Here's how the part is built. I have some questions about the finished solid (model axes, mm). A direction names the side the tool comes from. Coordinates: 2 decimals unless noted, no trailing zeros. Write each loop counter-clockwise with the first axis right and the second up, starting at its lowest first coordinate (ties: lowest second). Pieces come first, ordered by that corner, then holes.
Item 1: Please list where these lines run through material, in increasing order: line 1 (X direction, y = 18, z = 37.65); line 2 (Y direction, x = 24, z = 36.85); line 3 (X direction, y = -13, z = 12.5).
Item 2: I want a section at B-B (z = 25.2). Please give me the cut outline in (x, y).
Item 3: If we mould it in two halves opening along Y, with no side actions, what happens to faces 4 (the face through (-23.8, 17.92, 34.63)), 5 (the face through (32.5, 0, 19)), 6 (the face through (-35.95, 0.78, 31.15))? For each: pulls with the +Y half, pulls with the -Y half, needs draft (parallel to the pull), parting line crosses it, or undercut.
Item 4: I want a section at A-A (y = 0). Please give me the cut outline in (x, z), and give its area (3 significant figures).
Item 5: For faces 1 (the face through (-25.19, -17.62, 37.35)), 2 (the face through (0, -32.5, 19)), 3 (the face through (-22, 15, 0)), which set-ups out of +Z, -Z, +X, -X, +Y, -Y let a thin tool reach every point of the face, with its end or its side?
Item 6: I want a section at D-D (y = -14.5). Please give me the cut outline in (x, z).
Item 7: I'm going to push flat-ended pins straight in: P1, Ø2, axis at x = -24, y = -18, coming from the -Z side; P2, Ø2, axis at x = -24, y = 18, coming from the +Z side; P3, Ø1.5, axis at x = 13, y = 5.5, coming from the -Z side. Where does each tip first touch, or does it pass through?
Item 8: I want a section at C-C (x = -5.5). Please give me the cut outline in (y, z).
from build123d import *

# Parameters (mm, degrees)
SCHIZZO1_W                   = 65
SCHIZZO1_H                   = 65
ESTRUSIONE_ESTRUSIONE1_DEPTH = 39.5
SCHIZZO14_R                  = 6
ESTRUSIONE_ESTRUSIONE2_DEPTH = 7
FORO_FILETTATO_M3_1_D        = 2.5
FORO_FILETTATO_M3_1_DEPTH    = 4.248924226
FORO_FILETTATO_M3_1_TIP      = 0.751075774


with BuildPart() as part:
    # Schizzo1 → Estrusione-Estrusione1 (new body)
    with BuildSketch(Plane.XY):
        Rectangle(SCHIZZO1_W, SCHIZZO1_H)
    extrude(amount=ESTRUSIONE_ESTRUSIONE1_DEPTH)

    # Schizzo2 → Rivoluzione1 (revolve)
    with BuildSketch(Plane(origin=(0, 0, 0), x_dir=(1, 0, 0), z_dir=(0, 1, 0))):
        with BuildLine():
            Line((0, 0), (0, 20.5))
            Line((0, 20.5), (12.479983974, 20.5))
            ThreePointArc((12.479983974, 20.5), (20.922710333, 11.757558943), (24, 0))
            Line((24, 0), (0, 0))
        make_face()
    revolve(axis=Axis((0, 0, 0), (0, 0, -1)))

    # Schizzo14 → Estrusione-Estrusione2 (add)
    with BuildSketch(Plane.ZY.offset(32.5)):
        with Locations(Location((25.2, 0, 0), (0, 0, 270))):
            Circle(SCHIZZO14_R)
    extrude(amount=ESTRUSIONE_ESTRUSIONE2_DEPTH)

    # Foro filettato M3-1
    with Locations(Plane(origin=(-24, 18, 39.5), x_dir=(1, 0, 0), z_dir=(0, 0, 1))):
        with Locations((0, 0), (0, -36), (48, 0), (48, -36)):
            Hole(FORO_FILETTATO_M3_1_D / 2, depth=FORO_FILETTATO_M3_1_DEPTH)
            with Locations((0, 0, -(FORO_FILETTATO_M3_1_DEPTH + FORO_FILETTATO_M3_1_TIP / 2))):  # 118° drill point
                Cone(0, FORO_FILETTATO_M3_1_D / 2, FORO_FILETTATO_M3_1_TIP, mode=Mode.SUBTRACT)


solid = part.part
Answer:
1. line 1: x = -32.5 to -25.25, -22.75 to 22.75, 25.25 to 32.5
1. line 2: y = -32.5 to -19.25, -16.75 to 16.75, 19.25 to 32.5
1. line 3: x = -32.5 to 32.5
2. outline: (-39.5, -6) - (-32.5, -6) - (-32.5, -32.5) - (32.5, -32.5) - (32.5, 32.5) - (-32.5, 32.5) - (-32.5, 6) - (-39.5, 6) - close
3. face 4: undercut
3. face 5: needs draft
3. face 6: parting line crosses it
4. outline: (-39.5, 19.2) - (-32.5, 19.2) - (-32.5, 0) - (-24, 0) arc R24 ccw to (-12.48, -20.5) - (12.48, -20.5) arc R24 ccw to (24, 0) - (32.5, 0) - (32.5, 39.5) - (-32.5, 39.5) - (-32.5, 31.2) - (-39.5, 31.2) - close
4. area: 3,500 mm2
5. face 1: +Z
5. face 2: +Z, -Z, +X, -X, -Y
5. face 3: -Z
6. outline: (-32.5, 0) - (-19.12, 0) arc R19.12 ccw to (19.12, 0) - (32.5, 0) - (32.5, 39.5) - (-32.5, 39.5) - close
7. P1: stops at z = 0
7. P2: stops at z = 35.1
7. P3: stops at z = -19.93
8. outline: (-32.5, 0) - (-23.36, 0) arc R23.36 ccw to (-11.2, -20.5) - (11.2, -20.5) arc R23.36 ccw to (23.36, 0) - (32.5, 0) - (32.5, 39.5) - (-32.5, 39.5) - close
